Build history of the part. All positions in model axes, mm. Coordinates: 2 decimals unless noted, no trailing zeros. Write each loop counter-clockwise with the first axis right and the second up, starting at its lowest first coordinate (ties: lowest second). Pieces come first, ordered by that corner, then holes.
```python
from build123d import *

# Parameters (mm, degrees)
F0_W     = 30
F0_H     = 20
F1_DEPTH = 3.175
F2_R     = 1.5
F3_DEPTH = 25
F4_R     = 1


# Not quite as in the source:
# - a length typed as a fraction of an inch, garbled in the dataset ("3 / 203.2 mm" for 3/8 in), is restored


with BuildPart() as f1:
    # F0 (on Top) → F1 (new body)
    with BuildSketch(Plane.XY):
        with Locations((15, 10)):
            Rectangle(F0_W, F0_H)
    extrude(amount=F1_DEPTH)

    # F2 (on face) → F3 (cut)
    with BuildSketch(Plane.XY.offset(3.175)):
        with Locations((5, 16)):
            Circle(F2_R)
        with Locations((5, 4)):
            Circle(F2_R)
    extrude(amount=-F3_DEPTH, mode=Mode.SUBTRACT)

    # F4
    f4_edges = [f1.edges().sort_by_distance(p)[0] for p in [
        (0, 20, 1.5875),
        (30, 20, 1.5875),
        (30, 0, 1.5875),
        (0, 0, 1.5875),
    ]]
    fillet(f4_edges, radius=F4_R)


solid = f1.part
```
1. Saw through at C-C on y = 4. List the corners of the cut face in (x, z) (3 decimals), plus the area to 3 significant figures.
Computed values:
outline: (0, 0) - (3.5, 0) - (3.5, 3.175) - (0, 3.175) - close; (6.5, 0) - (30, 0) - (30, 3.175) - (6.5, 3.175) - close
area: 85.7 mm2
2. Probe line 1 along Y through (x, z) = (5, 0.7); line 2 along Y through (x, z) = (6, 1.55). List the from-to ranges inside material, lowest first.
Computed values:
line 1: y = 0 to 2.5, 5.5 to 14.5, 17.5 to 20
line 2: y = 0 to 2.88, 5.12 to 14.88, 17.12 to 20
3. Saw through at A-A on z = 2.8. List the corners of the cut face in (x, y), plus the area to 3 significant figures.
Computed values:
outline: (0, 1) arc R1 ccw to (1, 0) - (29, 0) arc R1 ccw to (30, 1) - (30, 19) arc R1 ccw to (29, 20) - (1, 20) arc R1 ccw to (0, 19) - close; hole circle Ø3 at (5, 4); hole circle Ø3 at (5, 16)
area: 585 mm2
4. Saw through at B-B on x = 5. List the corners of the cut face in (y, z) (3 decimals).
Computed values:
outline: (0, 0) - (2.5, 0) - (2.5, 3.175) - (0, 3.175) - close; (5.5, 0) - (14.5, 0) - (14.5, 3.175) - (5.5, 3.175) - close; (17.5, 0) - (20, 0) - (20, 3.175) - (17.5, 3.175) - close
5. Flat gauge pins, fed straight in: pin 1 (3.5 mm diameter, centred on x = 5, y = 16, fed in from -Z); pin 2 (2.5 mm diameter, centred on x = 5, y = 4, fed in from +Z). Where does each tip first touch, or does it go through?
Computed values:
pin 1: stops at z = 0
pin 2: passes through
6. Mould opens along X. For faces 1 (the face through (29.699, 0.285, 1.61)), 2 (the face through (15, 0, 2)), 3 (the face through (6.386, 15.425, 1.61)) say: +X half, -X half, draft (parallel to the pull), parting line (faces both ways), or undercut.
Computed values:
face 1: +X half
face 2: draft
face 3: undercut
